Input: dimensioned drawing with shaded views. Units: mm. Origin: part minimum x, y, z. A direction names the side the tool comes from. Round coordinates to 2 decimals unless told otherwise and drop trailing zeros. Write each loop counter-clockwise with the first axis right and the second up, starting at its lowest first coordinate (ties: lowest second). Pieces come first, ordered by that corner, then holes. Notation, with made-up numbers: M 57,85.25 L 76,85.25 A23 cw 76,117.25 Z; hole C 26.5,27.25 d2. An arc over 180 degrees is marked long. Put each result on its own line as item: value. Start each with the question number.
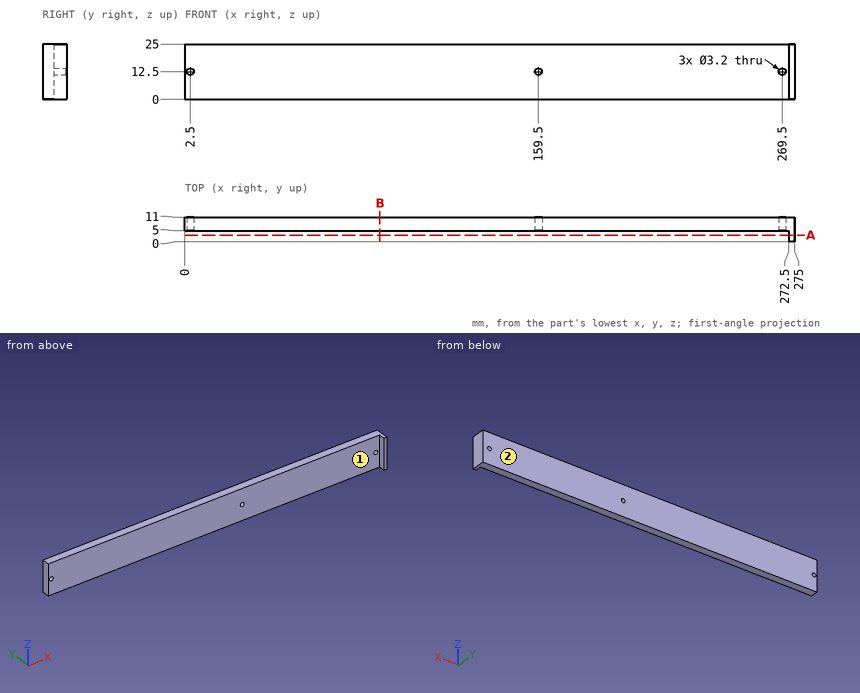
1) First-contact query: pin 1 (4 mm diameter, centred on x = 269.5, z = 12.5, fed in from -Y); pin 2 (3 mm diameter, centred on y = 3, z = 6.5, fed in from -X). Flat tips, straight axial feed; report the tip coordinate or a pass-through.
2) Section A-A, the plane y = 3. Output: boundary loops of the cut face in (x, z), and give its area (3 significant figures).
3) Access query for the marked faces 1 and 2. Directions: +Z, -Z, +X, -X, +Y, -Y. A direction counts if a zero-diameter tool reaches every point of the face in a straight line with its end or side. Return the directions, or none.
4) Section B-B, the plane x = 88. Output: boundary loops of the cut face in (y, z).
5) Ray query, probe 1 along X at (y, z) = (6.6, 12.5); probe 2 along Z at (x, y) = (269.5, 8.3); probe 3 along Y at (x, z) = (37, 8.5). Return the intervals inside material, ascending.
Solved:
1. pin 1: stops at y = 5
1. pin 2: stops at x = 272.5
2. outline: M 272.5,0 L 275,0 L 275,25 L 272.5,25 Z
2. area: 62.5 mm2
3. face 1: +Z, -Z, -X, -Y
3. face 2: +Z, -Z, +X, -X, +Y
4. outline: M 5,0 L 11,0 L 11,25 L 5,25 Z
5. probe 1: x = 0 to 0.9, 4.1 to 157.9, 161.1 to 267.9, 271.1 to 275
5. probe 2: z = 0 to 10.9, 14.1 to 25
5. probe 3: y = 5 to 11
